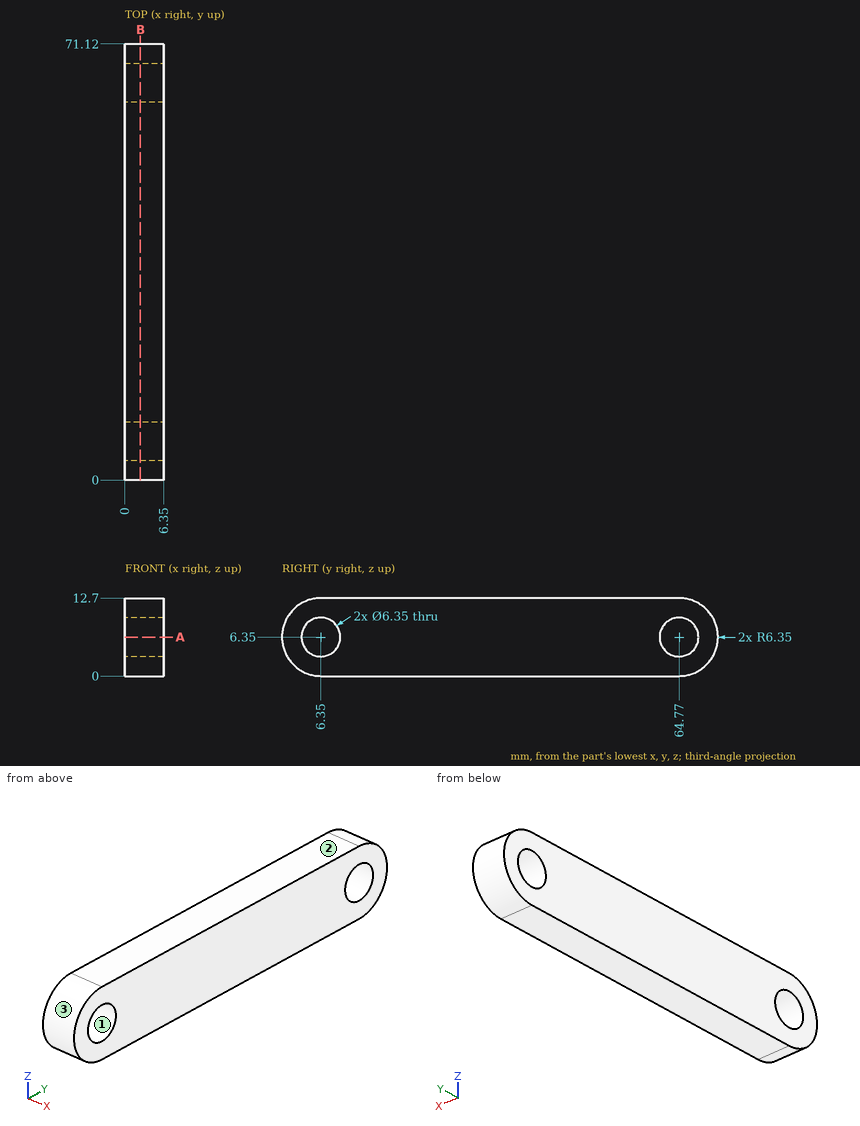
Study the drawing (mm; zero at the part's minimum x, y, z) and answer. Coordinates: 2 decimals unless noted, no trailing zeros. Write each loop counter-clockwise with the first axis right and the second up, starting at its lowest first coordinate (ties: lowest second). Pieces come first, ordered by that corner, then holes.
Q1. Find the intervals of material crossed by line 1 along Z through (x, y) = (2, 64.77) (3 decimals); line 2 along Y through (x, z) = (2, 8.5); line 3 along Y through (x, z) = (3.25, 5.75), in increasing order.
Returned:
line 1: z = 0 to 3.175, 9.525 to 12.7
line 2: y = 0.38 to 4.01, 8.69 to 62.43, 67.11 to 70.74
line 3: y = 0.03 to 3.23, 9.47 to 61.65, 67.89 to 71.09
Q2. Section B-B, the plane x = 2.5 is taken. Write down the section's boundary in (y, z) (3 decimals).
Returned:
outline: (6.35, 0) - (64.77, 0) arc R6.35 ccw to (64.77, 12.7) - (6.35, 12.7) arc R6.35 ccw to start; hole circle Ø6.35 at (6.35, 6.35); hole circle Ø6.35 at (64.77, 6.35)
Q3. Given P1, Ø2, axis at x = 4.5, z = 10.5, coming from the +Y side, flat-ended and moving along its own axis, determine where the tip first touches the part or whether it passes through.
Returned:
P1: stops at y = 70.28
Q4. The mould has two halves that part along Z. Classify the marked faces 1, 2 and 3: released by +Z, released by -Z, zero draft, split by the parting line, or undercut.
Returned:
face 1: undercut
face 2: released by +Z
face 3: split by the parting line
Q5. Section A-A, the plane z = 6.35 is taken. Write down the section's boundary in (x, y) (3 decimals), then the cut area to 3 significant figures.
Returned:
outline: (0, 0) - (6.35, 0) - (6.35, 3.175) - (0, 3.175) - close; (0, 9.525) - (6.35, 9.525) - (6.35, 61.595) - (0, 61.595) - close; (0, 67.945) - (6.35, 67.945) - (6.35, 71.12) - (0, 71.12) - close
area: 371 mm2
